from build123d import *

# Parameters (mm, degrees)
F0_W     = 41
F0_H     = 41
F1_DEPTH = 600
F2_W     = 6
F2_H     = 68
F3_DEPTH = 20
F4_W     = 6
F4_H     = 68
F5_DEPTH = 20


with BuildPart() as f1:
    # F0 (on Top) → F1 (new body)
    with BuildSketch(Plane.XY):
        with Locations((4.776136, -3.508085)):
            Rectangle(F0_W, F0_H)
    extrude(amount=F1_DEPTH)

    # F2 (on face) → F3 (cut)
    with BuildSketch(Plane(origin=(-15.723864, 0, 0), x_dir=(0, -1, 0), z_dir=(-1, 0, 0))):
        with Locations((8.508085, 46)):
            Rectangle(F2_W, F2_H)
    extrude(amount=-F3_DEPTH, mode=Mode.SUBTRACT)

    # F4 (on face) → F5 (cut)
    with BuildSketch(Plane(origin=(0, 16.991915, 0), x_dir=(-1, 0, 0), z_dir=(0, 1, 0))):
        with Locations((-9.776136, 46)):
            Rectangle(F4_W, F4_H)
    extrude(amount=-F5_DEPTH, mode=Mode.SUBTRACT)


solid = f1.part
Could you check a few things on this model? Use its own coordinates, in mm. A direction names the side the tool comes from. Give positions to 0.01 mm unless a question says otherwise; leave off trailing zeros. Order: outer loops, then holes, each group sorted by start corner. A loop starts at its lowest first (then second) coordinate and runs counter-clockwise, first axis right, second up. Notation, with made-up numbers: M 15.25,64.5 L 34.25,64.5 A17 ccw 34.25,70.5 Z; hole C 26.25,-40 d8. An arc over 180 degrees is marked long. One line per question, with ' | ' between items.
1. For faces 4 (the face through (-6, -11.508, 46)), 5 (the face through (6.776, 7, 46)), 6 (the face through (4, 16.992, 296)), which set-ups out of +Z, -Z, +X, -X, +Y, -Y let a thin tool reach every point of the face, with its end or its side?
Results:
face 4: -X | face 5: +Y | face 6: +Z, -Z, +X, -X, +Y
2. I want a section at A-A (x = -6.5). List the corners of the cut face in (y, z) for me, and give its area (3 significant figures).
Results:
outline: M -24.01,0 L 16.99,0 L 16.99,600 L -24.01,600 Z; hole M -11.51,12 L -5.51,12 L -5.51,80 L -11.51,80 Z | area: 24,200 mm²
3. I'm going to push flat-ended pins straight in: pin 1 (3 mm diameter, centred on x = 9, z = 32.5, fed in from +Y); pin 2 (1.8 mm diameter, centred on y = -8.5, z = 31, fed in from -X). Where does each tip first touch, or does it pass through?
Results:
pin 1: y = -3.01 | pin 2: x = 4.28
4. If I drill on line 1 (Z direction, x = 12.5, y = 0.5); line 2 (X direction, y = 13, z = 74); line 3 (Y direction, x = -7.5, z = 47), over which ranges is the centre line in solid material (lowest first)?
Results:
line 1: 0 to 12, 80 to 600 | line 2: -15.72 to 6.78, 12.78 to 25.28 | line 3: -24.01 to -11.51, -5.51 to 16.99
5. I want a section at C-C (z = 55). List the corners of the cut face in (x, y) for me.
Results:
outline: M -15.72,-24.01 L 25.28,-24.01 L 25.28,16.99 L 12.78,16.99 L 12.78,-3.01 L 6.78,-3.01 L 6.78,16.99 L -15.72,16.99 L -15.72,-5.51 L 4.28,-5.51 L 4.28,-11.51 L -15.72,-11.51 Z
6. I want a section at B-B (y = 8). List the corners of the cut face in (x, z) for me, and give its area (3 significant figures).
Results:
outline: M -15.72,0 L 25.28,0 L 25.28,600 L -15.72,600 Z; hole M 6.78,12 L 12.78,12 L 12.78,80 L 6.78,80 Z | area: 24,200 mm²
7. We'd pull the mould along Z, two halves only. Please class faces 1 (the face through (25.276, -4, 296)), 2 (the face through (4, -3, 0)), 3 (the face through (12.776, 7, 46)): +Z half, -Z half, draft (parallel to the pull), parting line (faces both ways), or undercut.
Results:
face 1: draft | face 2: -Z half | face 3: undercut
